Autodesk Inventor part; units mm, degrees
ref_plane "YZ Plane" through (0, 0, 0) normal (1, 0, 0) x (0, 1, 0)
ref_plane "XZ Plane" through (0, 0, 0) normal (0, 1, 0) x (-1, 0, 0)
ref_plane "XY Plane" through (0, 0, 0) normal (0, 0, 1) x (1, 0, 0)
sketch "Sketch1" plane through (0, 0, 0) normal (0, 0, 1) x (1, 0, 0)
  circle A0 centre (0, 0) radius 3.175
  line L0 (-1.508, 2.794) -> (1.508, 2.794)
  line L1 (-3.175, 0) -> (0, 0)
  line L2 (0, 0) -> (3.175, 0)
  line L3 (-1.508, -2.794) -> (1.508, -2.794)
  circle A1 centre (0, 0) radius 7.9375
  arc A2 (-4.892, 13.4239) -> (-4.892, -13.4239) centre (0, 0) ccw
  circle A3 centre (0, 10.0965) radius 1.905 construction
  circle A4 centre (0, 10.0965) radius 3.3274 construction
  circle A5 centre (0, 0) radius 10.0965
  line L4 (0, 0) -> (0, 10.0965) construction
  line L5 (0, -10.0965) -> (0, 0) construction
  line L6 (-4.892, 13.4239) -> (4.892, 13.4239)
  arc A6 (4.892, 13.4239) -> (-4.892, 13.4239) centre (0, 0) ccw
  circle A7 centre (0, -10.0965) radius 3.3274 construction
  line L7 (-4.892, -13.4239) -> (4.892, -13.4239)
  arc A8 (4.892, -13.4239) -> (4.892, 13.4239) centre (0, 0) ccw
  arc A9 (-4.892, -13.4239) -> (4.892, -13.4239) centre (0, 0) ccw
  dimension "d0" = 6.35
  dimension "d1" = 5.588
  dimension "d2" = 15.875
  dimension "d4" = 3.81
  dimension "d5" = 6.6548
  dimension "d7" = 2.159
  dimension "d8" = 14.2875
extrude "Extrusion1" add sketch "Sketch1" along normal blind 15.494 contours L6 A8 L7 A2 | A6 L6 | L7 A9 | A5
extrude "Extrusion2" add sketch "Sketch1" against normal blind 3.175 contours L0 A0 | A0 L3 | A1 | A5
extrude "Extrusion3" add sketch "Sketch1" along normal blind 3.175 contours L2 L1 A0 L0 | A0 L3 L1 L2 | L0 A0 | A0 L3 | A1
hole "Hole1" at (0, 0, 0) direction (0, 0, 1) diameter 3.302 end through all
sketch "Sketch2" plane through (0, 0, 3.175) normal (0, 0, 1) x (1, 0, 0)
  circle A0 centre (0, 0) radius 7.9375
  circle A1 centre (0, 0) radius 3.429 construction
  circle A2 centre (0, 0) radius 5.715
  dimension "d22" = 6.858
  dimension "d23" = 11.43
extrude "Extrusion4" add sketch "Sketch2" along normal blind 7.3406
sketch "Sketch3" plane through (0, 0, 15.494) normal (0, 0, 1) x (1, 0, 0)
  point P0 (0, -10.0965)
  point P1 (0, 10.0965)
hole "Hole2" at (0, 10.0965, 15.494) at (0, -10.0965, 15.494) direction (0, 0, -1) diameter 2.6416 depth 9.525 tip angle 118
chamfer "Chamfer2" distance 3.175 angle 45 1 edges at (-4.892, 13.4239, 0)
extrude "Extrusion5" cut sketch "Sketch1" along normal up to surface (15.494 mm away) contours A6 L6 | L7 A9
sketch "Sketch4" plane through (0, 0, 0) normal (0, 0, -1) x (-1, 0, 0)
  circle A0 centre (0, 0) radius 1.651
  line L0 (1.508, 2.794) -> (-1.508, 2.794)
  arc A1 (-1.508, 2.794) -> (-1.508, -2.794) centre (0, 0) ccw
  line L1 (-1.508, -2.794) -> (1.508, -2.794)
  arc A2 (1.508, -2.794) -> (1.508, 2.794) centre (0, 0) ccw
extrude "Extrusion6" add sketch "Sketch4" along normal blind 0.254
properties part number "Pnuematic Connector"
Part model, mm, in its own coordinate system. A direction names the side the tool comes from. Round coordinates to 2 decimals unless told otherwise and drop trailing zeros. Order: outer loops, then holes, each group sorted by start corner. A loop starts at its lowest first (then second) coordinate and runs counter-clockwise, first axis right, second up. Notation, with made-up numbers: M 27,-23.5 L 52,-23.5 A20 cw 52,-12.5 Z; hole C 44,-17.75 d9. An arc over 180 degrees is marked long. Answer in a Markdown table with one row per item. Add a question column.
Q1. Cut at A-A on z = 11.5. Give the cut face in (x, y) (1 decimal).
Q2. 3-axis set-ups, long thin cutter, end or side, ignore diameter. For faces 1 (the face through (0.804, 11.145, 10.665)), 2 (the face through (-3.175, 0.048, -1.694)), 3 (the face through (14.285, 0.244, 9.248)): which of +Z, -Z, +X, -X, +Y, -Y reach the whole face in a straight line?
Q3. Pin check, flat tips, straight feed: pin 1 (4.5 mm diameter, centred on x = 0, y = 0, fed in from -Z); pin 2 (1 mm diameter, centred on x = -4, z = 1, fed in from +Y); pin 3 (5 mm diameter, centred on x = 8.5, z = 11.5, fed in from -Y). Stop position of each tip, or through.
Q4. Wall check: L1, parallel to Y at x = 0, z = 12.65; L2, parallel to Y at x = 0, z = 10 (3 decimals); L3, parallel to Y at x = 0, z = 5 (3 decimals). Give the ranges that are in metal, low to high. Write a range as from..to.
Q5. Cut at C-C on z = 1. Give the cut face in (x, y) (1 decimal), and give its area (3 significant figures).
Q6. Cut at B-B on y = 0. Give the cut face in (x, z) (1 decimal).
Q7. Mould opens along X. For faces 4 (the face through (-2.4, 2.4, -3.175)), 5 (the face through (-1.456, 0.779, 1.485)), 6 (the face through (4.336, 10.447, 0.199)), 7 (the face through (-14.285, -0.244, 9.248)) say: +X half, -X half, draft (parallel to the pull), parting line (faces both ways), or undercut.
Established:
| question | item | result |
|---|---|---|
| 1 | outline | M -4.9,-13.4 L 4.9,-13.4 A14.3 ccw 4.9,13.4 L -4.9,13.4 A14.3 ccw Z; hole C 0,0 d15.9; hole C 0,-10.1 d2.6; hole C 0,10.1 d2.6 |
| 2 | face 1 | +Z |
| 2 | face 2 | -Z |
| 2 | face 3 | +Z, -Z, +X |
| 3 | pin 1 | stops at z = -0.25 |
| 3 | pin 2 | stops at y = 11.99 |
| 3 | pin 3 | stops at y = -12.97 |
| 4 | L1 | y = -13.42..-11.42, -8.78..-7.94, 7.94..8.78, 11.42..13.42 |
| 4 | L2 | y = -13.424..-11.417, -8.776..-5.715, 5.715..8.776, 11.417..13.424 |
| 4 | L3 | y = -13.424..-5.715, 5.715..13.424 |
| 5 | outline | C 0,0 d24.2; hole C 0,0 d3.3 |
| 5 | area | 452 mm2 |
| 6 | outline | M -14.3,3.2 L -11.1,0 L -10.1,0 L -10.1,-3.2 L -3.2,-3.2 L -3.2,-0.3 L -1.7,-0.3 L -1.7,3.2 L -5.7,3.2 L -5.7,10.5 L -7.9,10.5 L -7.9,15.5 L -14.3,15.5 Z; M 1.7,-0.3 L 3.2,-0.3 L 3.2,-3.2 L 10.1,-3.2 L 10.1,0 L 11.1,0 L 14.3,3.2 L 14.3,15.5 L 7.9,15.5 L 7.9,10.5 L 5.7,10.5 L 5.7,3.2 L 1.7,3.2 Z |
| 7 | face 4 | draft |
| 7 | face 5 | undercut |
| 7 | face 6 | parting line |
| 7 | face 7 | -X half |
